```python
from build123d import *

# Parameters (mm, degrees)
SKETCH1_W           = 110.8
SKETCH1_H           = 82
BOSS_EXTRUDE1_DEPTH = 5
CUT_EXTRUDE1_DEPTH  = 10
SKETCH3_W           = 34.2
SKETCH3_H           = 5.2
CUT_EXTRUDE2_DEPTH  = 10
CUT_EXTRUDE3_DEPTH  = 10


with BuildPart() as part:
    # Sketch1 → Boss-Extrude1 (new body)
    with BuildSketch(Plane.XY):
        Rectangle(SKETCH1_W, SKETCH1_H)
    extrude(amount=BOSS_EXTRUDE1_DEPTH)

    # Sketch2 → Cut-Extrude1 (cut)
    with BuildSketch(Plane.XY.offset(5)):
        Polygon((41, -32.6), (41, -22.6), (45.4, -22.6), (45.4, -32.6), (46.9, -32.6), (46.9, -36), (45.4, -36), (45.4, -41), (41, -41), (41, -36), (39.5, -36), (39.5, -32.6), align=None)
        Polygon((-41, 32.6), (-41, 22.6), (-45.4, 22.6), (-45.4, 32.6), (-46.9, 32.6), (-46.9, 36), (-45.4, 36), (-45.4, 41), (-41, 41), (-41, 36), (-39.5, 36), (-39.5, 32.6), align=None)
        Polygon((45.4, 22.6), (45.4, 32.6), (46.9, 32.6), (46.9, 36), (45.4, 36), (45.4, 41), (41, 41), (41, 36), (39.5, 36), (39.5, 32.6), (41, 32.6), (41, 22.6), align=None)
        Polygon((-45.4, -22.6), (-45.4, -32.6), (-46.9, -32.6), (-46.9, -36), (-45.4, -36), (-45.4, -41), (-41, -41), (-41, -36), (-39.5, -36), (-39.5, -32.6), (-41, -32.6), (-41, -22.6), align=None)
    extrude(amount=-CUT_EXTRUDE1_DEPTH, mode=Mode.SUBTRACT)

    # Sketch3 → Cut-Extrude2 (cut)
    with BuildSketch(Plane.XY.offset(5)):
        with Locations((0, -38.4)):
            Rectangle(SKETCH3_W, SKETCH3_H)
    extrude(amount=-CUT_EXTRUDE2_DEPTH, mode=Mode.SUBTRACT)

    # Sketch4 → Cut-Extrude3 (cut)
    with BuildSketch(Plane.XY.offset(5)):
        with BuildLine():
            Line((35, -14), (14.6, -14))
            ThreePointArc((14.6, -14), (11.6, -11), (14.6, -8))
            Line((14.6, -8), (35, -8))
            ThreePointArc((35, -8), (38, -11), (35, -14))
        make_face()
        with BuildLine():
            Line((-14.6, -8), (-35, -8))
            ThreePointArc((-35, -8), (-38, -11), (-35, -14))
            Line((-35, -14), (-14.6, -14))
            ThreePointArc((-14.6, -14), (-11.6, -11), (-14.6, -8))
        make_face()
    extrude(amount=-CUT_EXTRUDE3_DEPTH, mode=Mode.SUBTRACT)


solid = part.part
```
Geometry check sheet. Reference: the model listing, model coordinates, mm. A direction names the side the tool comes from. Coordinates: 2 decimals unless noted, no trailing zeros. Write each loop counter-clockwise with the first axis right and the second up, starting at its lowest first coordinate (ties: lowest second). Pieces come first, ordered by that corner, then holes. Notation, with made-up numbers: M -39,82 L -19,82 A27 cw -19,102 Z; hole C -25.75,25.25 d6. An arc over 180 degrees is marked long. Use one line per item in the form item = value. Start each with the question number.
1) Go/stop test with a flat-tipped pin: pin 1 Ø8 at (x, y) = (39, -9.5) entering from -Z. Record where the tip stops, or that it passes through.
2) Set-up check for faces 1 (the flat face through (50, -41, 2)), 2 (the flat face through (25, -8, 3)), 3 (the flat face through (41, -28, 3)), 4 (the flat face through (45.4, 28, 3)): record each of +Z, -Z, +X, -X, +Y, -Y from which the full face is reachable in a straight line by a thin tool's end or side.
3) Section check A-A on y = 30.5. Enter the section's corners in (x, z).
4) Release check for a two-part mould opening along X. For faces 5 (the flat face through (29, -41, 2)), 6 (the flat face through (-39.5, -34, 3)) record: pulls with the +X half, pulls with the -X half, needs draft (parallel to the pull), parting line crosses it, or undercut.
5) Section check B-B on x = -32. Enter the section's corners in (y, z), and give its area (3 significant figures).
6) Section check C-C on y = -11. Enter the section's corners in (x, z).
7) Thickness scan on probe 1 along X at (y, z) = (33.5, 4.55); probe 2 along Y at (x, z) = (40, 1.5); probe 3 along X at (y, z) = (24.5, 0.55). Record the ranges inside material, lowest first. Write a range as from..to.
8) Section check D-D on z = 3.15. State how many separate pieces and enclosed holes the cut face has, and give its area (3 significant figures).
Responses:
q1.pin_1 = 0
q2.face_1 = +Z, -Z, +X, -X, -Y
q2.face_2 = +Z, -Z
q2.face_3 = +Z, -Z, -Y
q2.face_4 = +Z, -Z, +Y
q3.outline = M -55.4,0 L -45.4,0 L -45.4,5 L -55.4,5 Z; M -41,0 L 41,0 L 41,5 L -41,5 Z; M 45.4,0 L 55.4,0 L 55.4,5 L 45.4,5 Z
q4.face_5 = needs draft
q4.face_6 = undercut
q5.outline = M -41,0 L -14,0 L -14,5 L -41,5 Z; M -8,0 L 41,0 L 41,5 L -8,5 Z
q5.area = 380 mm2
q6.outline = M -55.4,0 L -38,0 L -38,5 L -55.4,5 Z; M -11.6,0 L 11.6,0 L 11.6,5 L -11.6,5 Z; M 38,0 L 55.4,0 L 55.4,5 L 38,5 Z
q7.probe_1 = -55.4..-46.9, -39.5..39.5, 46.9..55.4
q7.probe_2 = -41..-36, -32.6..32.6, 36..41
q7.probe_3 = -55.4..-45.4, -41..41, 45.4..55.4
q8.separate_pieces = 1
q8.enclosed_holes = 2
q8.area = 8,240 mm2
